Geometry: final body of the model. Coordinates: model frame, mm. A direction names the side the tool comes from. Give positions to 0.01 mm unless a question says otherwise; leave off trailing zeros. Loops run counter-clockwise (first coordinate to the right, second up) from the corner with the lowest first, then second, coordinate; pieces in that order, holes last. Notation, with made-up numbers: (74.25, 79) -> (120.25, 79) arc R15 ccw to (120.25, 83) -> close; hole circle Ø5 at (7.5, 41.25). An arc over 180 degrees is marked (long way). One line per item, written item: value. Start each with the question number.
from build123d import *

# Parameters (mm, degrees)
SKETCH1_R           = 47.5
BOSS_EXTRUDE1_DEPTH = 220
SKETCH2_R           = 25
BOSS_EXTRUDE2_DEPTH = 280
CHAMFER1_SIZE       = 5


with BuildPart() as part:
    # Sketch1 → Boss-Extrude1 (new body, symmetric)
    with BuildSketch(Plane(origin=(0, 0, 0), x_dir=(0, 0, -1), z_dir=(1, 0, 0))):
        Circle(SKETCH1_R)
    extrude(amount=BOSS_EXTRUDE1_DEPTH, both=True)

    # Sketch2 → Boss-Extrude2 (add, symmetric)
    with BuildSketch(Plane(origin=(0, 0, 0), x_dir=(0, 0, -1), z_dir=(1, 0, 0))):
        Circle(SKETCH2_R)
    extrude(amount=BOSS_EXTRUDE2_DEPTH, both=True)

    # Chamfer1
    chamfer1_edges = [part.edges().sort_by_distance(p)[0] for p in [
        (-280, 0, 25),
        (280, 0, 25),
    ]]
    chamfer(chamfer1_edges, length=CHAMFER1_SIZE)


solid = part.part
Item 1: Section C-C, the plane x = 73. Output: boundary loops of the cut face in (y, z).
Item 2: Pin query (flat end, axial travel): pin 1 (4 mm diameter, centred on x = 61.5, y = -33, fed in from -Z); pin 2 (8 mm diameter, centred on y = -21, z = -34, fed in from +X); pin 3 (5 mm diameter, centred on x = 91, y = -32.5, fed in from +Z). Return the tip coordinate at first contact, or that it passes through.
Item 3: Section A-A, the plane y = 0. Output: boundary loops of the cut face in (x, z), then the cut area to 4 significant figures.
Item 4: Section D-D, the plane z = 38.5. Output: boundary loops of the cut face in (x, y), then the cut area to 3 significant figures.
Item 5: Access query for faces 1 (the face through (-220, -20, -20)), 2 (the face through (220, -20, -20)), 3 (the face through (-280, 0, 0)). Directions: +Z, -Z, +X, -X, +Y, -Y. A direction counts if a zero-diameter tool reaches every point of the face in a straight line with its end or side. Return the directions, or none.
Item 6: Ray query, line 1 along X through (y, z) = (-8, -28); line 2 along Y through (x, z) = (49, 6.5); line 3 along Y through (x, z) = (106, -26.5). Return the intervals inside material, ascending. Write a range as [from, to].
Geometry check:
1. outline: circle Ø95 at (0, 0)
2. pin 1: stops at z = -35.99
2. pin 2: stops at x = 220
2. pin 3: stops at z = 36.83
3. outline: (-280, -20) -> (-275, -25) -> (-220, -25) -> (-220, -47.5) -> (220, -47.5) -> (220, -25) -> (275, -25) -> (280, -20) -> (280, 20) -> (275, 25) -> (220, 25) -> (220, 47.5) -> (-220, 47.5) -> (-220, 25) -> (-275, 25) -> (-280, 20) -> close
3. area: 47,750 mm2
4. outline: (-220, -27.82) -> (220, -27.82) -> (220, 27.82) -> (-220, 27.82) -> close
4. area: 24,500 mm2
5. face 1: -X
5. face 2: +X
5. face 3: +Z, -Z, -X, +Y, -Y
6. line 1: x = [-220, 220]
6. line 2: y = [-47.05, 47.05]
6. line 3: y = [-39.42, 39.42]
